Input: part model. Units: mm. Frame: model coordinates. A direction names the side the tool comes from. Coordinates: 2 decimals unless noted, no trailing zeros. Loops run counter-clockwise (first coordinate to the right, second up) from the corner with the lowest first, then second, coordinate; pieces in that order, holes last. Notation, with made-up numbers: (-23.5, 3) - (13.5, 3) arc R25 cw to (13.5, 27) - close; hole circle Ø6 at (23.25, -18.5). An arc over 180 degrees is marked (long way). Use one line per item in the form item = value.
from build123d import *

# Parameters (mm, degrees)
SKETCH4_W           = 4
SKETCH4_H           = 4.5
BOSS_EXTRUDE1_DEPTH = 5.5
SKETCH5_R           = 0.5
BOSS_EXTRUDE2_DEPTH = 5
SKETCH6_R           = 1.75
CUT_EXTRUDE1_DEPTH  = 5
SKETCH7_R           = 1
CUT_EXTRUDE2_DEPTH  = 2


with BuildPart() as part:
    # Sketch4 → Boss-Extrude1 (new body)
    with BuildSketch(Plane(origin=(0, 0, 0), x_dir=(1, 0, 0), z_dir=(0, 1, 0))):
        Rectangle(SKETCH4_W, SKETCH4_H)
    extrude(amount=BOSS_EXTRUDE1_DEPTH)

    # Sketch5 → Boss-Extrude2 (add)
    with BuildSketch(Plane.XY.offset(2.25)):
        with Locations(Location((0, 2.5, 0), (0, 0, 180))):
            Circle(SKETCH5_R)
    extrude(amount=BOSS_EXTRUDE2_DEPTH)

    # Sketch6 → Cut-Extrude1 (cut)
    with BuildSketch(Plane(origin=(0, 5.5, 0), x_dir=(1, 0, 0), z_dir=(0, 1, 0))):
        with Locations(Location((0, 0, 0), (0, 0, 270))):
            Circle(SKETCH6_R)
    extrude(amount=-CUT_EXTRUDE1_DEPTH, mode=Mode.SUBTRACT)

    # Sketch7 → Cut-Extrude2 (cut)
    with BuildSketch(Plane(origin=(0, 0, -2.25), x_dir=(-1, 0, 0), z_dir=(0, 0, -1))):
        with Locations((0, 3.5)):
            Circle(SKETCH7_R)
    extrude(amount=-CUT_EXTRUDE2_DEPTH, mode=Mode.SUBTRACT)


solid = part.part
Q1. Cut plane C-C, the plane z = 0. Return loops of the section in (x, y).
Check values:
outline = (-2, 0) - (2, 0) - (2, 5.5) - (1.75, 5.5) - (1.75, 0.5) - (-1.75, 0.5) - (-1.75, 5.5) - (-2, 5.5) - close
Q2. Cut plane B-B, the plane y = 4.8. Return loops of the section in (x, z), then the cut area to 3 significant figures.
Check values:
outline = (-2, -2.25) - (2, -2.25) - (2, 2.25) - (-2, 2.25) - close; hole circle Ø3.5 at (0, 0)
area = 8.38 mm²
Q3. Cut plane A-A, the plane x = 0. Return loops of the section in (y, z).
Check values:
outline = (0, -2.25) - (2.5, -2.25) - (2.5, -1.75) - (0.5, -1.75) - (0.5, 1.75) - (5.5, 1.75) - (5.5, 2.25) - (3, 2.25) - (3, 7.25) - (2, 7.25) - (2, 2.25) - (0, 2.25) - close; (4.5, -2.25) - (5.5, -2.25) - (5.5, -1.75) - (4.5, -1.75) - close
Q4. Pull-direction query (X, two-part tool) for faces 5 (the flat face through (2, 3, 0)), 6 (the flat face through (0, 0.5, 0)), 7 (the flat face through (0, 2.5, 7.25)); classes: pulls with the +X half, pulls with the -X half, needs draft (parallel to the pull), parting line crosses it, or undercut.
Check values:
face_5 = pulls with the +X half
face_6 = undercut
face_7 = needs draft
Q5. Cut plane D-D, the plane y = 3.5. Return loops of the section in (x, z), then the cut area to 3 significant figures.
Check values:
outline = (-2, -2.25) - (-1, -2.25) - (-1, -1.44) arc R1.75 cw (long way) to (1, -1.44) - (1, -2.25) - (2, -2.25) - (2, 2.25) - (-2, 2.25) - close
area = 7.18 mm²
Q6. Ray query, line 1 along Y through (x, z) = (0, -1.9); line 2 along X through (y, z) = (3.5, -2.05); line 3 along X through (y, z) = (2.2, 0). Return the intervals inside material, ascending. Write a range as [from, to].
Check values:
line_1 = [0, 2.5], [4.5, 5.5]
line_2 = [-2, -1], [1, 2]
line_3 = [-2, -1.75], [1.75, 2]
Q7. Set-up query: faces 1 (the cylindrical face through (-0.954, 3.8, -1.939)), 2 (the flat face through (-2, 3, 0)), 3 (the cylindrical face through (-0.67, 3.035, 1.617)), 4 (the cylindrical face through (0, 2, 5)). Return all of +Z, -Z, +X, -X, +Y, -Y with unobstructed straight access to the full face (end or side cutting, diameter ignored); none if empty.
Check values:
face_1 = -Z
face_2 = +Z, -Z, -X, +Y, -Y
face_3 = +Y
face_4 = +Z
Q8. First-contact query: P1, Ø2, axis at x = -1, y = 2.5, coming from the +Z side; P2, Ø1, axis at x = 1, y = 3.5, coming from the +Z side. Flat tips, straight axial feed; report the tip coordinate or a pass-through.
Check values:
P1 = 7.25
P2 = 2.25
